from build123d import *

# Parameters (mm, degrees)
EXTRUDE_3_DEPTH = 1


with BuildPart() as part:
    # 草图1 → 凸台-拉伸3 (new body)
    with BuildSketch(Plane.XY):
        with BuildLine():
            Line((-30.25, 25.75), (-30.25, -25.75))
            ThreePointArc((-30.25, -25.75), (-28.858757211, -29.108757211), (-25.5, -30.5))
            Line((-25.5, -30.5), (25.5, -30.5))
            ThreePointArc((25.5, -30.5), (28.858757211, -29.108757211), (30.25, -25.75))
            Line((30.25, -25.75), (30.25, 25.75))
            ThreePointArc((30.25, 25.75), (28.858757211, 29.108757211), (25.5, 30.5))
            Line((25.5, 30.5), (-25.5, 30.5))
            ThreePointArc((-25.5, 30.5), (-28.858757211, 29.108757211), (-30.25, 25.75))
        make_face()
        with BuildLine():
            Line((-2.5, -25), (2.5, -25))
            ThreePointArc((2.5, -25), (3.5, -26), (2.5, -27))
            Line((2.5, -27), (-2.5, -27))
            ThreePointArc((-2.5, -27), (-3.5, -26), (-2.5, -25))
        make_face(mode=Mode.SUBTRACT)
    extrude(amount=EXTRUDE_3_DEPTH)


solid = part.part
Geometry check sheet. Reference: the model listing, model coordinates, mm. Give positions to 0.01 mm unless a question says otherwise; leave off trailing zeros. Order: outer loops, then holes, each group sorted by start corner. A loop starts at its lowest first (then second) coordinate and runs counter-clockwise, first axis right, second up.
1) Cross-section at A-A (x = 1.5). Record the boundary of the cut face in (y, z), then the cut area to 3 significant figures.
Results are:
outline: (-30.5, 0) - (-27, 0) - (-27, 1) - (-30.5, 1) - close; (-25, 0) - (30.5, 0) - (30.5, 1) - (-25, 1) - close
area: 59.0 mm2
2) Gauge pin test, flat end, axial feed: pin 1 (1.5 mm diameter, centred on x = -15.5, y = -14.5, fed in from -Z). Record the tip position at first contact, or that the pin passes through.
Results are:
pin 1: stops at z = 0
3) Material ranges on probe 1 along Y at (x, z) = (27, 0.15); probe 2 along Y at (x, z) = (-26.5, 0.55), recorded low to high.
Results are:
probe 1: y = -30.26 to 30.26
probe 2: y = -30.39 to 30.39
